Check sheet for the modelled part. Datum: model origin and axes. Units: mm. Face numbers are marked on the shaded views. A direction names the side the tool comes from. Round coordinates to 2 decimals unless told otherwise and drop trailing zeros. Write each loop counter-clockwise with the first axis right and the second up, starting at its lowest first coordinate (ties: lowest second). Pieces come first, ordered by that corner, then holes. Notation, with made-up numbers: (24.25, 52.25) - (32.25, 52.25) arc R18 cw to (32.25, 63.25) - close; hole circle Ø8 at (13.5, 33). An arc over 180 degrees is marked (long way). Answer as a JSON object with one key per item and string values. Group by question number.
Item 1: Release check for a two-part mould opening along Z. For the marked faces 1, 2, 3 and 4 record: pulls with the +Z half, pulls with the -Z half, needs draft (parallel to the pull), parting line crosses it, or undercut.
Item 2: Sectioned sample at A-A on z = 0. Record the boundary of the cut face in (x, y), plus the area to 3 significant figures.
Item 3: Sectioned sample at D-D on x = 2.5. Record the boundary of the cut face in (y, z).
Item 4: Thickness scan on line 1 (Z direction, x = 10.75, y = 0); line 2 (Z direction, x = 4.75, y = 0); line 3 (X direction, y = -10.5, z = -0.25). Record the ranges inside material, lowest first.
Item 5: Set-up check for the marked faces 5 and 6: record each of +Z, -Z, +X, -X, +Y, -Y from which the full face is reachable in a straight line by a thin tool's end or side.
Item 6: Gauge pin test, flat ends, axial feed: P1, Ø3, axis at y = 0, z = 2.5, coming from the +X side; P2, Ø6, axis at x = 5, y = -5, coming from the -Z side; P3, Ø3.5, axis at y = 0, z = 0, coming from the -X side; P4, Ø1, axis at x = 7.5, y = -5, coming from the -Z side. Record the tip position at first contact, or that the pin passes through.
Item 7: Sectioned sample at C-C on x = 8.5. Record the boundary of the cut face in (y, z).
Autodesk Inventor part; units mm, degrees
ref_plane "YZ Plane" through (0, 0, 0) normal (1, 0, 0) x (0, 1, 0)
ref_plane "XZ Plane" through (0, 0, 0) normal (0, 1, 0) x (-1, 0, 0)
ref_plane "XY Plane" through (0, 0, 0) normal (0, 0, 1) x (1, 0, 0)
sketch "Skizze1" plane through (0, 0, 0) normal (0, 0, 1) x (1, 0, 0)
  line L0 (0, 0) -> (0, 12)
  line L1 (0, 12) -> (5, 12)
  line L2 (5, 12) -> (5, 9.5)
  line L3 (5, 9.5) -> (10.9, 9.5)
  line L4 (10.9, 9.5) -> (10.9, 5)
  line L5 (0, 0) -> (10.1, 0)
  line L6 (10.9, 5) -> (10.1, 5)
  line L7 (10.1, 5) -> (10.1, 0)
  dimension "d0" = 19
  dimension "d1" = 24
  dimension "d2" = 5.9
  dimension "d3" = 5
  dimension "d12" = 10
  dimension "d13" = 5.1
revolve "Umdrehung1" add sketch "Skizze1" angle 360 about axis through (0, 0, 0) along (1, 0, 0)
sketch "Skizze2" plane through (0, 0, 0) normal (-1, 0, 0) x (0, 0, 1)
  point P0 (0, 0)
  point P1 (0, 0)
hole "Bohrung1" at (0, 0, 0) direction (1, 0, 0) diameter 4.134 depth 14.2 tip angle 118
feature "Verdickung1" [suppressed]
thicken "Verdickung2" operation add thickness 0.1 both sides no extend neighbours yes toward (0, 0.9967573, -0.0804666) faces at (10.3667, 4.9838, -0.4023)
properties part number "SpringCompensation_Innside_DrivenPart"
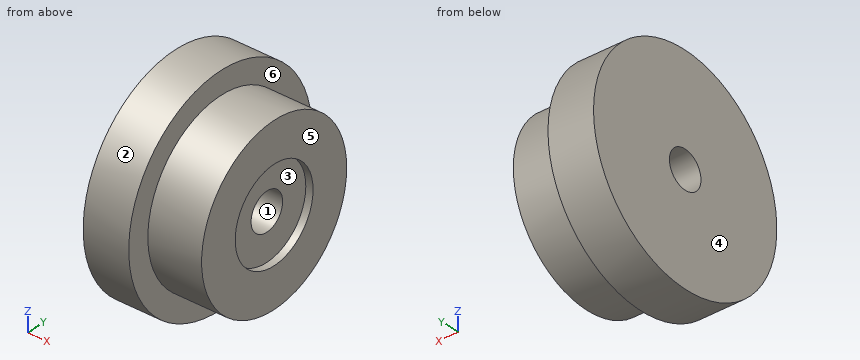
Completed:
{
 "1": {"face 1": "undercut", "face 2": "parting line crosses it", "face 3": "undercut", "face 4": "needs draft"},
 "2": {"outline": "(0, -12) - (5, -12) - (5, -9.5) - (10.9, -9.5) - (10.9, -5.1) - (10.1, -5.1) - (10.1, -2.07) - (0, -2.07) - close; (0, 2.07) - (10.1, 2.07) - (10.1, 5.1) - (10.9, 5.1) - (10.9, 9.5) - (5, 9.5) - (5, 12) - (0, 12) - close", "area": "182 mm²"},
 "3": {"outline": "circle Ø24 at (0, 0); hole circle Ø4.13 at (0, 0)"},
 "4": {"line 1": "-9.5 to -5.1, 5.1 to 9.5", "line 2": "-12 to -2.07, 2.07 to 12", "line 3": "0 to 5"},
 "5": {"face 5": "+Z, -Z, +X, +Y, -Y", "face 6": "+X"},
 "6": {"P1": "x = 10.1", "P2": "z = -11.83", "P3": "through", "P4": "z = -8.37"},
 "7": {"outline": "circle Ø19 at (0, 0); hole circle Ø4.13 at (0, 0)"}
}
